```python
from build123d import *

# Parameters (mm, degrees)
SKETCH1_W           = 10
SKETCH1_H           = 8
SKETCH1_W_2         = 22
SKETCH1_H_2         = 1
BOSS_EXTRUDE1_DEPTH = 3
SKETCH2_W           = 10
SKETCH2_H           = 8
BOSS_EXTRUDE2_DEPTH = 3


with BuildPart() as part:
    # Sketch1 → Boss-Extrude1 (new, symmetric)
    with BuildSketch(Plane(origin=(0, 0, 0), x_dir=(1, 0, 0), z_dir=(0, 1, 0))):
        with Locations((5, 0)):
            Rectangle(SKETCH1_W, SKETCH1_H)
        with Locations((-11, 0)):
            Rectangle(SKETCH1_W_2, SKETCH1_H_2)
    extrude(amount=BOSS_EXTRUDE1_DEPTH, both=True)

    # Sketch2 → Boss-Extrude2 (add)
    with BuildSketch(Plane(origin=(0, 3, 0), x_dir=(1, 0, 0), z_dir=(0, 1, 0))):
        with Locations((5, 0)):
            Rectangle(SKETCH2_W, SKETCH2_H)
    extrude(amount=BOSS_EXTRUDE2_DEPTH)


solid = part.part
```
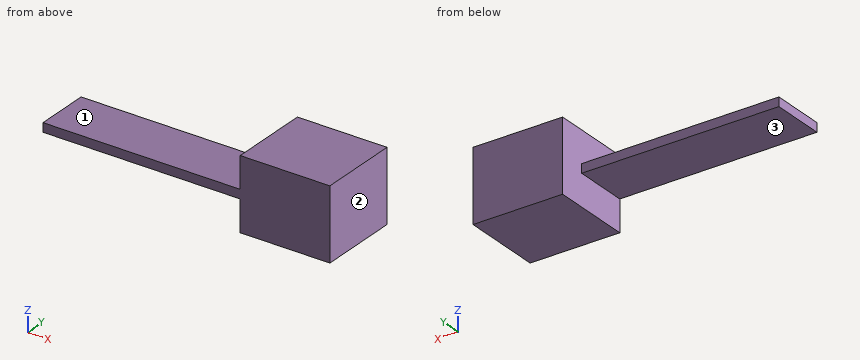
CAD build for the part. Positions are in the model's coordinates, mm. Face numbers are marked on the shaded views. A direction names the side the tool comes from. Coordinates: 2 decimals unless noted, no trailing zeros. Write each loop counter-clockwise with the first axis right and the second up, starting at its lowest first coordinate (ties: lowest second). Pieces come first, ordered by that corner, then holes.
(1) Cut at A-A, the plane y = -1. List the corners of the cut face in (x, z).
(2) Drill centre lines: probe 1 along Z at (x, y) = (-17, 2.5); probe 2 along X at (y, z) = (-0.5, -2.25); probe 3 along Y at (x, z) = (-9, 0.25). Where is each one in solid material? Low to high.
(3) Cut at B-B, the plane x = -16.5. List the corners of the cut face in (y, z).
(4) Cut at C-C, the plane z = -2. List the corners of the cut face in (x, y).
(5) Flat gauge pins, fed straight in: pin 1 (3 mm diameter, centred on x = -7, y = -1, fed in from +Z); pin 2 (1.8 mm diameter, centred on x = -6.5, y = 0, fed in from -Z); pin 3 (2 mm diameter, centred on y = 2.5, z = 2.5, fed in from -X). Where does each tip first touch, or does it go through?
(6) 3-axis set-ups, long thin cutter, end or side, ignore diameter. For the marked faces 1, 2 and 3: which of +Z, -Z, +X, -X, +Y, -Y reach the whole face in a straight line?
Geometry says:
1. outline: (-22, -0.5) - (0, -0.5) - (0, -4) - (10, -4) - (10, 4) - (0, 4) - (0, 0.5) - (-22, 0.5) - close
2. probe 1: z = -0.5 to 0.5
2. probe 2: x = 0 to 10
2. probe 3: y = -3 to 3
3. outline: (-3, -0.5) - (3, -0.5) - (3, 0.5) - (-3, 0.5) - close
4. outline: (0, -3) - (10, -3) - (10, 6) - (0, 6) - close
5. pin 1: stops at z = 0.5
5. pin 2: stops at z = -0.5
5. pin 3: stops at x = 0
6. face 1: +Z, -X, +Y, -Y
6. face 2: +Z, -Z, +X, +Y, -Y
6. face 3: -Z, -X, +Y, -Y
